Answer from the drawing. Dimensions are ordinates in mm from the lowest x, y and z of the part. A direction names the side the tool comes from. Give positions to 0.01 mm unless a question says otherwise; leave off trailing zeros. Loops run counter-clockwise (first coordinate to the right, second up) from the corner with the lowest first, then second, coordinate; pieces in that order, holes last.
(1) Find section A-A, the plane y = 7. Write down the section's boundary in (x, z), then the cut area to 3 significant figures.
(2) Find section B-B, the plane x = 25. Write down the section's boundary in (y, z), then the cut area to 3 significant figures.
(3) Find section C-C, the plane z = 30. Write down the section's boundary in (x, y).
(4) Determine the mould class of the marked faces 1, 2, 3 and 4 for opening direction X: pulls with the +X half, pulls with the -X half, needs draft (parallel to the pull), parting line crosses it, or undercut.
(5) Which of the six approach directions +Z, -Z, +X, -X, +Y, -Y give full straight-line access (tool end or side, diameter ignored) to the marked faces 5, 6, 7 and 8?
(6) Straight lines are drawn through the part: probe 1 along Z at (x, y) = (20.5, 28); probe 2 along Y at (x, z) = (25, 10); probe 3 along X at (y, z) = (22, 31). For each, find the intervals that lie inside material, in ascending order.
(7) Each of these flat-tipped pins is pushed along its axis until it touches: P1, Ø12, axis at x = 33.5, y = 30, coming from the -Z side; P2, Ø2, axis at y = 15, z = 29.5, coming from the -X side; P3, Ø1.5, axis at y = 31, z = 12, coming from the +X side; P4, Ø6, axis at x = 25, y = 22, coming from the +Z side. Where does it stop, or does it pass through?
(8) Find section D-D, the plane y = 21. Write down the section's boundary in (x, z), then the cut area to 3 significant figures.
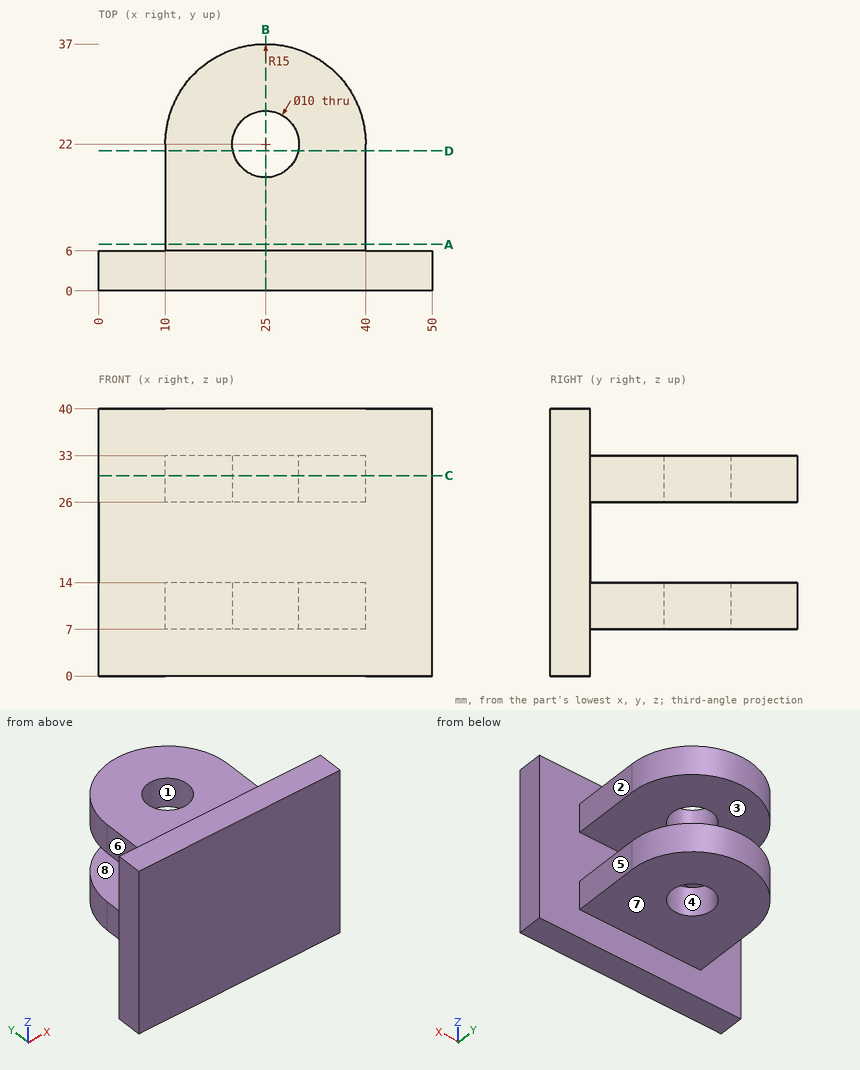
Entries:
1. outline: (10, 7) - (40, 7) - (40, 14) - (10, 14) - close; (10, 26) - (40, 26) - (40, 33) - (10, 33) - close
1. area: 420 mm2
2. outline: (0, 0) - (6, 0) - (6, 7) - (17, 7) - (17, 14) - (6, 14) - (6, 26) - (17, 26) - (17, 33) - (6, 33) - (6, 40) - (0, 40) - close; (27, 7) - (37, 7) - (37, 14) - (27, 14) - close; (27, 26) - (37, 26) - (37, 33) - (27, 33) - close
2. area: 534 mm2
3. outline: (0, 0) - (50, 0) - (50, 6) - (40, 6) - (40, 22) arc R15 ccw to (10, 22) - (10, 6) - (0, 6) - close; hole circle Ø10 at (25, 22)
4. face 1: undercut
4. face 2: pulls with the +X half
4. face 3: needs draft
4. face 4: undercut
5. face 5: +Z, -Z, +X, +Y
5. face 6: +Z, -Z, -X, +Y
5. face 7: -Z, +X, -X, +Y
5. face 8: +X, -X, +Y
6. probe 1: z = 7 to 14, 26 to 33
6. probe 2: y = 0 to 17, 27 to 37
6. probe 3: x = 10 to 20, 30 to 40
7. P1: stops at z = 7
7. P2: stops at x = 10
7. P3: stops at x = 37.53
7. P4: passes through
8. outline: (10, 7) - (20.1, 7) - (20.1, 14) - (10, 14) - close; (10, 26) - (20.1, 26) - (20.1, 33) - (10, 33) - close; (29.9, 7) - (40, 7) - (40, 14) - (29.9, 14) - close; (29.9, 26) - (40, 26) - (40, 33) - (29.9, 33) - close
8. area: 283 mm2
